Verification items for the finished model (mm, model axes). Coordinates: 2 decimals unless noted, no trailing zeros. Write each loop counter-clockwise with the first axis right and the second up, starting at its lowest first coordinate (ties: lowest second). Pieces come first, ordered by that corner, then holes. Notation, with made-up numbers: M -3.5,31 L 20.5,31 A27 cw 20.5,60 Z; hole C 2,-39 d9. An arc over 180 degrees is marked long. Answer in a Markdown table with one row per item.
from build123d import *

# Parameters (mm, degrees)
F1_DEPTH = 23.6
F2_W     = 149.606
F2_H     = 93.3704
F3_DEPTH = 1


with BuildPart() as f1:
    # F0 (on Front) → F1 (new body)
    with BuildSketch(Plane.XZ):
        with BuildLine():
            Line((91.125, 66.675), (-91.125, 66.675))
            ThreePointArc((-91.125, 66.675), (-105.267136, 60.817136), (-111.125, 46.675))
            Line((-111.125, 46.675), (-111.125, -46.675))
            ThreePointArc((-111.125, -46.675), (-105.267136, -60.817136), (-91.125, -66.675))
            Line((-91.125, -66.675), (91.125, -66.675))
            ThreePointArc((91.125, -66.675), (105.267136, -60.817136), (111.125, -46.675))
            Line((111.125, -46.675), (111.125, 46.675))
            ThreePointArc((111.125, 46.675), (105.267136, 60.817136), (91.125, 66.675))
        make_face()
    extrude(amount=F1_DEPTH)

    # F2 (on face) → F3 (cut)
    with BuildSketch(Plane.XZ.offset(23.6)):
        Rectangle(F2_W, F2_H)
    extrude(amount=-F3_DEPTH, mode=Mode.SUBTRACT)


solid = f1.part
1) Thickness scan on L1, parallel to Y at x = 31, z = -27.5; L2, parallel to Z at x = -92, y = -3; L3, parallel to X at y = -20, z = -59.5. Record the ranges inside material, lowest first. Write a range as [from, to].
Response values:
| item | result |
|---|---|
| L1 | y = [-22.6, 0] |
| L2 | z = [-66.66, 66.66] |
| L3 | x = [-106.47, 106.47] |
2) Depth check by flat-ended pin: pin 1 (6 mm diameter, centred on x = 35, z = -23.5, fed in from -Y). Enter the tip coordinate at first touch or a pass-through.
Response values:
| item | result |
|---|---|
| pin 1 | stops at y = -22.6 |
3) Sectioned sample at C-C (z = 55.5). Record the cut outline in (x, y).
Response values:
| item | result |
|---|---|
| outline | M -109.07,-23.6 L 109.07,-23.6 L 109.07,0 L -109.07,0 Z |
4) Sectioned sample at B-B (z = -9.5). Record the cut outline in (x, y) (3 decimals), then the cut area to 3 significant figures.
Response values:
| item | result |
|---|---|
| outline | M -111.125,-23.6 L -74.803,-23.6 L -74.803,-22.6 L 74.803,-22.6 L 74.803,-23.6 L 111.125,-23.6 L 111.125,0 L -111.125,0 Z |
| area | 5,100 mm² |
5) Sectioned sample at A-A (x = -10). Record the cut outline in (y, z) (3 decimals), then the cut area to 3 significant figures.
Response values:
| item | result |
|---|---|
| outline | M -23.6,-66.675 L 0,-66.675 L 0,66.675 L -23.6,66.675 L -23.6,46.685 L -22.6,46.685 L -22.6,-46.685 L -23.6,-46.685 Z |
| area | 3,050 mm² |
6) Release check for a two-part mould opening along X. For faces 1 (the face through (-1, -22.6, 1)), 2 (the face through (-111.125, -12, 1)), 3 (the face through (-1, -12, -66.675)), 4 (the face through (111.125, -12, -1)) record: +X half, -X half, draft (parallel to the pull), parting line (faces both ways), or undercut.
Response values:
| item | result |
|---|---|
| face 1 | undercut |
| face 2 | -X half |
| face 3 | draft |
| face 4 | +X half |
